from build123d import *

# Parameters (mm, degrees)
F0_W     = 44.1192735617
F0_H     = 11.1166509635
F1_DEPTH = 5.14096
F2_R     = 5.08
F3_R     = 5.08
F4_W     = 1.4028784636
F4_H     = 5.165201461
F4_W_2   = 0.8638333529
F4_W_3   = 0.9213921431
F4_W_4   = 1.4403553497
F4_W_5   = 1.3910879198
F4_W_6   = 1.2432860676
F4_W_7   = 0.8935106736
F4_W_8   = 1.0018550383
F4_W_9   = 1.3910882691
F4_W_10  = 1.1940188706
F4_W_11  = 1.3041589975
F4_W_12  = 0.9969494123
F4_W_13  = 0.9587099776
F4_W_14  = 0.8777634058
F5_DEPTH = 0.3302


# Not quite as in the source:
# - a feature names something its author has since deleted; it is built from what else it names


with BuildPart() as f1:
    # F0 (on Right) → F1 (new body, symmetric)
    with BuildSketch(Plane.YZ):
        Rectangle(F0_W, F0_H)
    extrude(amount=F1_DEPTH, both=True)

    # F2
    f2_edges = [f1.edges().sort_by_distance(p)[0] for p in [
        (5.14096, 22.059637, 0),
        (5.14096, -22.059637, 0),
    ]]
    fillet(f2_edges, radius=F2_R)

    # F3
    f3_edges = [f1.edges().sort_by_distance(p)[0] for p in [
        (-2.54, 22.059637, 5.558325),
    ]]
    fillet(f3_edges, radius=F3_R)

    # F4 (on face) → F5 (join)
    with BuildSketch(Plane.YZ.offset(5.14096)):
        Polygon((9.4375805929, -5.5583254817), (11.1789442599, -5.5583254817), (11.1789442599, 0.4704763523), (8.4788706154, 0.4704763523), (7.0501212031, 0.4704763523), (4.8823622055, 0.4704763523), (3.2565433066, 0.4704763523), (1.4336550375, 0.4704763523), (0, 0.4704763523), (-1.3253106736, 0.4704763523), (-3.0003967695, 0.4704763523), (-4.8232846893, 0.4704763523), (-6.695440039, 0.4704763523), (-11.1789442599, 0.4704763523), (-11.1789442599, -5.5583254817), (-8.9124655351, -5.5583254817), (-6.695440039, -5.5583254817), (-4.8232846893, -5.5583254817), (-3.0003967695, -5.5583254817), (-1.3253106736, -5.5583254817), (0, -5.5583254817), (1.4336550375, -5.5583254817), (3.2565433066, -5.5583254817), (4.8823622055, -5.5583254817), (7.0501212031, -5.5583254817), (8.4788706154, -5.5583254817), align=None)
        with Locations((-10.0457047669, -2.5439243782)):
            Rectangle(F4_W, F4_H, mode=Mode.SUBTRACT)
        with Locations((-8.4805488586, -2.5439243782)):
            Rectangle(F4_W_2, F4_H, mode=Mode.SUBTRACT)
        with Locations((-7.1561361106, -2.5439243782)):
            Rectangle(F4_W_3, F4_H, mode=Mode.SUBTRACT)
        with Locations((-5.5434623642, -2.5439243782)):
            Rectangle(F4_W_4, F4_H, mode=Mode.SUBTRACT)
        with Locations((-3.6959407294, -2.5439243782)):
            Rectangle(F4_W_5, F4_H, mode=Mode.SUBTRACT)
        with Locations((-1.9469537074, -2.5439243782)):
            Rectangle(F4_W_6, F4_H, mode=Mode.SUBTRACT)
        with Locations((-0.4467553368, -2.5439243782)):
            Rectangle(F4_W_7, F4_H, mode=Mode.SUBTRACT)
        with Locations((0.9327275184, -2.5439243782)):
            Rectangle(F4_W_8, F4_H, mode=Mode.SUBTRACT)
        with Locations((2.5609991721, -2.5439243782)):
            Rectangle(F4_W_9, F4_H, mode=Mode.SUBTRACT)
        with Locations((4.2853527702, -2.5439243782)):
            Rectangle(F4_W_10, F4_H, mode=Mode.SUBTRACT)
        with Locations((5.9662417043, -2.5439243782)):
            Rectangle(F4_W_11, F4_H, mode=Mode.SUBTRACT)
        with Locations((7.5485959092, -2.5439243782)):
            Rectangle(F4_W_12, F4_H, mode=Mode.SUBTRACT)
        with Locations((8.9582256041, -2.5439243782)):
            Rectangle(F4_W_13, F4_H, mode=Mode.SUBTRACT)
        with Locations((10.3082622958, -2.5439243782)):
            Rectangle(F4_W_14, F4_H, mode=Mode.SUBTRACT)
    extrude(amount=F5_DEPTH)


solid = f1.part
Can you work these out from the model? Positions are in its coordinate system, mm. A direction names the side the tool comes from. Give positions to 0.01 mm unless a question says otherwise; leave off trailing zeros. Order: outer loops, then holes, each group sorted by start corner. A loop starts at its lowest first (then second) coordinate and runs counter-clockwise, first axis right, second up. Notation, with made-up numbers: M 62.5,56 L 88.5,56 A19 cw 88.5,92 Z; hole C 4,74 d5. An arc over 180 degrees is marked long. Use a Markdown table: item, result. Add a question column.
Item 1: Will these pins go through, and if not, where does the flat tip stop? pin 1 (6 mm diameter, centred on y = 16, z = -0.5, fed in from +X); pin 2 (1.5 mm diameter, centred on y = 13.5, z = 2.5, fed in from +X).
Item 2: Suppose I cut it at C-C (z = 1.5). List the corners of the cut face in (x, y) for me, then the cut area to 3 significant figures.
Item 3: We'd pull the mould along Y, two halves only. Please class faces 3 (the flat face through (5.141, 4, -3)), 4 (the cylindrical face through (3.613, -20.611, -2.498)), 5 (the flat face through (0, 0, -5.558)), 6 (the flat face through (5.141, -2, -3)): +Y half, -Y half, draft (parallel to the pull), parting line (faces both ways), or undercut.
Item 4: Suppose I cut it at B-B (x = -3.75). List the corners of the cut face in (y, z) for me, then the cut area to 3 significant figures.
Item 5: For faces 1 (the flat face through (5.141, 6, -3)), 2 (the flat face through (-5.141, 0, 0)), which set-ups out of +Z, -Z, +X, -X, +Y, -Y let a thin tool reach every point of the face, with its end or its side?
Item 6: Suppose I cut it at D-D (y = 13). List the corners of the cut face in (x, z) for me.
Item 7: If I drill on L1, parallel to X at y = 3, z = -3.25; L2, parallel to Z at x = -4, y = 19.5; L3, parallel to Y at x = -3.5, z = 3.5, over which ranges is the centre line in solid material (lowest first)? Write a range as [from, to].
Answer sheet:
| question | item | result |
|---|---|---|
| 1 | pin 1 | stops at x = 5.14 |
| 1 | pin 2 | stops at x = 4.98 |
| 2 | outline | M -5.14,-21.96 L 0.06,-21.96 A4.98 ccw 5.04,-16.98 L 5.04,16.98 A4.98 ccw 0.06,21.96 L -5.14,21.96 Z |
| 2 | area | 436 mm² |
| 3 | face 3 | undercut |
| 3 | face 4 | -Y half |
| 3 | face 5 | draft |
| 3 | face 6 | undercut |
| 4 | outline | M -22.06,-5.56 L 22.06,-5.56 L 22.06,0.48 A5.08 ccw 16.98,5.56 L -16.98,5.56 A5.08 ccw -22.06,0.48 Z |
| 4 | area | 479 mm² |
| 5 | face 1 | +X |
| 5 | face 2 | +Z, -Z, -X, +Y, -Y |
| 6 | outline | M -5.14,-5.56 L 5.14,-5.56 L 5.14,0.48 A5.08 ccw 0.06,5.56 L -5.14,5.56 Z |
| 7 | L1 | x = [-5.14, 5.14] |
| 7 | L2 | z = [-5.56, 4.89] |
| 7 | L3 | y = [-21.06, 21.06] |
